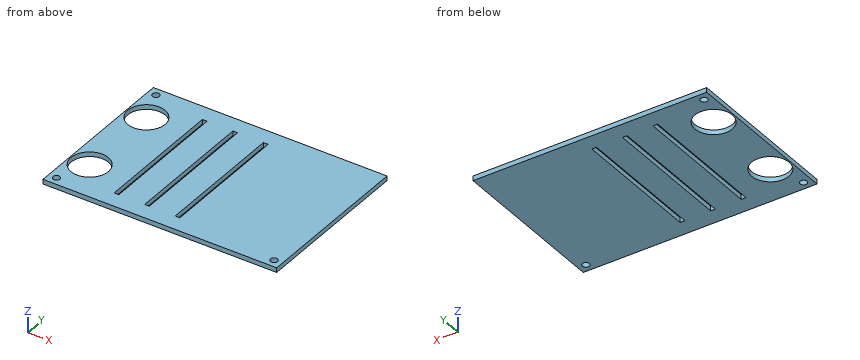
```python
from build123d import *

# Parameters (mm, degrees)
SKETCH_1_W      = 100
SKETCH_1_H      = 70
SKETCH_1_R      = 1.5
SKETCH_1_R_2    = 8
SKETCH_1_W_2    = 2
SKETCH_1_H_2    = 56
EXTRUDE_1_DEPTH = 2


with BuildPart() as part:
    # ｽｹｯﾁ1 → ﾎﾞｽ - 押し出し1 (new body)
    with BuildSketch(Plane.XY):
        with Locations((50, -35)):
            Rectangle(SKETCH_1_W, SKETCH_1_H)
        with Locations((3.45, -3.45)):
            Circle(SKETCH_1_R, mode=Mode.SUBTRACT)
        with Locations(Location((3.45, -66.55, 0), (0, 0, 180))):
            Circle(SKETCH_1_R, mode=Mode.SUBTRACT)
        with Locations((96.55, -66.55)):
            Circle(SKETCH_1_R, mode=Mode.SUBTRACT)
        with Locations((8.5, -17)):
            Circle(SKETCH_1_R_2, mode=Mode.SUBTRACT)
        with Locations(Location((8.5, -53, 0), (0, 0, 180))):
            Circle(SKETCH_1_R_2, mode=Mode.SUBTRACT)
        with Locations((52.84, -35)):
            Rectangle(SKETCH_1_W_2, SKETCH_1_H_2, mode=Mode.SUBTRACT)
        with Locations((39.76, -35)):
            Rectangle(SKETCH_1_W_2, SKETCH_1_H_2, mode=Mode.SUBTRACT)
        with Locations((26.7, -35)):
            Rectangle(SKETCH_1_W_2, SKETCH_1_H_2, mode=Mode.SUBTRACT)
    extrude(amount=EXTRUDE_1_DEPTH)


solid = part.part
```
Geometry check sheet. Reference: the model listing, model coordinates, mm. Give positions to 0.01 mm unless a question says otherwise; leave off trailing zeros. Write each loop counter-clockwise with the first axis right and the second up, starting at its lowest first coordinate (ties: lowest second). Pieces come first, ordered by that corner, then holes. Notation, with made-up numbers: (19, 3) - (75, 3) arc R32 cw to (75, 29) - close; hole circle Ø2 at (61.25, 69). An arc over 180 degrees is marked (long way). Use a Markdown table: item, result.
Q1. Section check D-D, the plane z = 1.35. Give the number of separate pieces and of enclosed holes in the cut face, then the cut area to 3 significant figures.
Computed:
| item | result |
|---|---|
| separate pieces | 1 |
| enclosed holes | 8 |
| area | 6,240 mm² |
Q2. Go/stop test with a flat-tipped pin: P1, Ø1.8, axis at x = 3.45, y = -3.45, coming from the -Z side. Record where the tip stops, or that it passes through.
Computed:
| item | result |
|---|---|
| P1 | passes through |
Q3. Section check C-C, the plane y = -66.55. Enter the section's corners in (x, z), then the cut area to 3 significant figures.
Computed:
| item | result |
|---|---|
| outline | (0, 0) - (1.95, 0) - (1.95, 2) - (0, 2) - close; (4.95, 0) - (95.05, 0) - (95.05, 2) - (4.95, 2) - close; (98.05, 0) - (100, 0) - (100, 2) - (98.05, 2) - close |
| area | 188 mm² |
Q4. Section check B-B, the plane x = 96.55. Enter the section's corners in (y, z).
Computed:
| item | result |
|---|---|
| outline | (-70, 0) - (-68.05, 0) - (-68.05, 2) - (-70, 2) - close; (-65.05, 0) - (0, 0) - (0, 2) - (-65.05, 2) - close |
Q5. Thickness scan on L1, parallel to X at y = -28, z = 1.5; L2, parallel to X at y = -53, z = 0.65; L3, parallel to Y at x = 8.5, z = 1.4. Record the ranges inside material, lowest first. Write a range as [from, to].
Computed:
| item | result |
|---|---|
| L1 | x = [0, 25.7], [27.7, 38.76], [40.76, 51.84], [53.84, 100] |
| L2 | x = [0, 0.5], [16.5, 25.7], [27.7, 38.76], [40.76, 51.84], [53.84, 100] |
| L3 | y = [-70, -61], [-45, -25], [-9, 0] |
Q6. Section check A-A, the plane y = -53. Enter the section's corners in (x, z), then the cut area to 3 significant figures.
Computed:
| item | result |
|---|---|
| outline | (0, 0) - (0.5, 0) - (0.5, 2) - (0, 2) - close; (16.5, 0) - (25.7, 0) - (25.7, 2) - (16.5, 2) - close; (27.7, 0) - (38.76, 0) - (38.76, 2) - (27.7, 2) - close; (40.76, 0) - (51.84, 0) - (51.84, 2) - (40.76, 2) - close; (53.84, 0) - (100, 0) - (100, 2) - (53.84, 2) - close |
| area | 156 mm² |
